from build123d import *

# Parameters (mm, degrees)
SKETCH_2_OUTSIDE_W   = 59.726
SKETCH_2_OUTSIDE_H   = 59.726
SKETCH_2_OUTSIDE_W_2 = 8
SKETCH_2_OUTSIDE_H_2 = 8
CUT_EXTRUDE_1_DEPTH  = 17
HOLE_WIZARD_M4_1_D   = 3.3


with BuildPart() as part:
    # 草图1 → 旋转1 (revolve)
    with BuildSketch(Plane.XY):
        Polygon((114, 0), (114, 5), (95.1, 5), (95.1, 4.8), (94, 4.8), (94, 5), (15, 5), (15, 6), (-15, 6), (-15, 5), (-94, 5), (-94, 4.8), (-95.1, 4.8), (-95.1, 5), (-114, 5), (-114, 0), align=None)
    revolve(axis=Axis((-114, 0, 0), (1, 0, 0)))

    # 草图2 outside → 切除-拉伸1 (cut)
    with BuildSketch(Plane(origin=(114, 0, 0), x_dir=(0, 0, -1), z_dir=(1, 0, 0))):
        Rectangle(SKETCH_2_OUTSIDE_W, SKETCH_2_OUTSIDE_H)
        Rectangle(SKETCH_2_OUTSIDE_W_2, SKETCH_2_OUTSIDE_H_2, mode=Mode.SUBTRACT)
    cut_extrude_1 = extrude(amount=-CUT_EXTRUDE_1_DEPTH, mode=Mode.SUBTRACT)

    # 镜向2: 切除-拉伸1 across plane
    add(cut_extrude_1.mirror(Plane(origin=(0, 0, 0), x_dir=(0, 0, 1), z_dir=(1, 0, 0))), mode=Mode.SUBTRACT)

    # M4 螺纹孔1 (through all)
    with Locations(Plane.XY.offset(4)):
        with Locations((109, 0), (-109, 0)):
            Hole(HOLE_WIZARD_M4_1_D / 2)


solid = part.part
The listing builds one solid part. Answer for the finished solid, in the listing's coordinates (mm). A direction names the side the tool comes from. Give positions to 0.01 mm unless a question says otherwise; leave off trailing zeros. Order: outer loops, then holes, each group sorted by start corner. A loop starts at its lowest first (then second) coordinate and runs counter-clockwise, first axis right, second up. Notation, with made-up numbers: (42, 27) - (85, 27) arc R30 ccw to (85, 59) - close; hole circle Ø6 at (85, 66.25). An arc over 180 degrees is marked (long way). One line per item, written item: value. Start each with the question number.
1) A cutting plane is placed at B-B on z = 0. State how many separate pieces and enclosed holes the cut face has, then the cut area to 3 significant figures.
2) The mould has two halves that part along X. Classify faces 1 (the face through (-94.56, 2.58, 4.05)), 2 (the face through (-106, 0, -4)), 3 (the face through (-15, -4, 4)): released by +X, released by -X, zero draft, split by the parting line, or undercut.
3) Given pin 1 Ø6.5 at (x, z) = (-107.5, -1) entering from +Y; pin 2 Ø6.5 at (x, y) = (105.5, -1.5) entering from +Z; pin 3 Ø3 at (x, z) = (107.5, 0.5) entering from -Y; pin 4 Ø1.1 at (y, z) = (1, -4.5) entering from -X, each flat-ended and moving along its own axis, determine where each tip first touches the part or whether it passes through.
4) A tool of negligible diameter and unlimited length cuts with its end or side. For faces 4 (the face through (-106, 4, 0)), 5 (the face through (-106, 0, 4)), 6 (the face through (106, 4, 0)), 7 (the face through (106, 0, -4)), 8 (the face through (101.006, -3.877, -3.157)), from which of +Z, -Z, +X, -X, +Y, -Y can it reach the whole face along a straight path? Write none if from no direction.
5) Find the intervals of material crossed by L1, parallel to Y at x = 109, z = 1.75; L2, parallel to X at y = -1, z = -2; L3, parallel to X at y = -1.5, z = 4.5, in increasing order.
6) A cutting plane is placed at A-A on x = -58.5. Give the vertices of the cut face in (y, z), then the cut area to 3 significant figures.
Answer sheet:
1. separate pieces: 1
1. enclosed holes: 2
1. area: 2,250 mm2
2. face 1: undercut
2. face 2: zero draft
2. face 3: released by -X
3. pin 1: stops at y = 4
3. pin 2: stops at z = 4
3. pin 3: stops at y = -4
3. pin 4: stops at x = -114
4. face 4: +Z, -Z, -X, +Y
4. face 5: +Z, -X, +Y, -Y
4. face 6: +Z, -Z, +X, +Y
4. face 7: -Z, +X, +Y, -Y
4. face 8: +X
5. L1: y = -4 to -1.65, 1.65 to 4
5. L2: x = -114 to -110.31, -107.69 to 107.69, 110.31 to 114
5. L3: x = -97 to 97
6. outline: circle Ø10 at (0, 0)
6. area: 78.5 mm2
